Design review of the part built by this model. Coordinates are the model's own, in mm. A direction names the side the tool comes from. Coordinates: 2 decimals unless noted, no trailing zeros. Write each loop counter-clockwise with the first axis right and the second up, starting at its lowest first coordinate (ties: lowest second). Pieces come first, ordered by that corner, then holes. Notation, with made-up numbers: (76.5, 77.25) - (84.5, 77.25) arc R16 ccw to (84.5, 108.25) - close; hole circle Ø5 at (5, 60.25). An arc over 180 degrees is marked (long way). Use a Markdown table: item, result.
from build123d import *

# Parameters (mm, degrees)
F0_W           = 5.9
F0_H           = 1.1
F1_DEPTH       = 2.9
F2_W           = 5.9
F2_H           = 1.85
F3_DEPTH       = 2
F5_D           = 3.2
F5_CSINK_D     = 5.6
F5_CSINK_ANGLE = 82
F6_DEPTH       = 1.1
F7_R           = 1
F8_W           = 3
F8_H           = 1.2
F9_DEPTH       = 2.6
F10_W          = 1.6
F10_H          = 2.7
F10_H_2        = 1.55
F11_DEPTH      = 3.5
F12_W          = 1.6
F12_H          = 1.35
F13_DEPTH      = 1.6
F15_DEPTH      = 2.8


with BuildPart() as f1:
    # F0 (on Top) → F1 (new body)
    with BuildSketch(Plane.XY):
        with BuildLine():
            Line((4.95, 1.6), (4.95, 0))
            Line((4.95, 0), (12.45, 0))
            Line((12.45, 0), (12.45, 1.6))
            Line((12.45, 1.6), (15.45, 1.6))
            Line((15.45, 1.6), (15.45, 0))
            Line((15.45, 0), (19.3, 0))
            Line((19.3, 0), (19.3, 1.1))
            Line((19.3, 1.1), (25.2, 1.1))
            Line((25.2, 1.1), (25.2, 0))
            Line((25.2, 0), (29.05, 0))
            Line((29.05, 0), (29.05, 1.6))
            Line((29.05, 1.6), (32.05, 1.6))
            Line((32.05, 1.6), (32.05, 0))
            Line((32.05, 0), (39.55, 0))
            Line((39.55, 0), (39.55, 1.6))
            Line((39.55, 1.6), (42.55, 1.6))
            Line((42.55, 1.6), (42.55, 0))
            Line((42.55, 0), (42.7, 0))
            ThreePointArc((42.7, 0), (43.9727922061, 0.5272077939), (44.5, 1.8))
            Line((44.5, 1.8), (44.5, 42.7))
            ThreePointArc((44.5, 42.7), (43.9727922061, 43.9727922061), (42.7, 44.5))
            Line((42.7, 44.5), (42.55, 44.5))
            Line((42.55, 44.5), (42.55, 42.9))
            Line((42.55, 42.9), (39.55, 42.9))
            Line((39.55, 42.9), (39.55, 44.5))
            Line((39.55, 44.5), (32.05, 44.5))
            Line((32.05, 44.5), (32.05, 42.9))
            Line((32.05, 42.9), (29.05, 42.9))
            Line((29.05, 42.9), (29.05, 44.5))
            Line((29.05, 44.5), (25.2, 44.5))
            Line((25.2, 44.5), (25.2, 43.4))
            Line((25.2, 43.4), (19.3, 43.4))
            Line((19.3, 43.4), (19.3, 44.5))
            Line((19.3, 44.5), (15.45, 44.5))
            Line((15.45, 44.5), (15.45, 42.9))
            Line((15.45, 42.9), (12.45, 42.9))
            Line((12.45, 42.9), (12.45, 44.5))
            Line((12.45, 44.5), (4.95, 44.5))
            Line((4.95, 44.5), (4.95, 42.9))
            Line((4.95, 42.9), (1.95, 42.9))
            Line((1.95, 42.9), (1.95, 44.5))
            Line((1.95, 44.5), (1.8, 44.5))
            ThreePointArc((1.8, 44.5), (0.5272077939, 43.9727922061), (0, 42.7))
            Line((0, 42.7), (0, 1.8))
            ThreePointArc((0, 1.8), (0.5272077939, 0.5272077939), (1.8, 0))
            Line((1.8, 0), (1.95, 0))
            Line((1.95, 0), (1.95, 1.6))
            Line((1.95, 1.6), (4.95, 1.6))
        make_face()
        with Locations((22.25, -0.55)):
            Rectangle(F0_W, F0_H)
        with Locations((22.25, 0.55)):
            Rectangle(F0_W, F0_H)
        with Locations((22.25, 43.95)):
            Rectangle(F0_W, F0_H)
        with Locations((22.25, 45.05)):
            Rectangle(F0_W, F0_H)
    extrude(amount=F1_DEPTH)

    # F2 (on face) → F3 (join)
    with BuildSketch(Plane(origin=(0, 0, 0), x_dir=(1, 0, 0), z_dir=(0, 0, -1))):
        with Locations((22.25, 0.175)):
            Rectangle(F2_W, F2_H)
        with BuildLine():
            Line((25.2, -0.75), (19.3, -0.75))
            Line((19.3, -0.75), (9.7372574326, -2.4247745488))
            ThreePointArc((9.7372574326, -2.4247745488), (4.9258838609, -4.9258838609), (2.4247745488, -9.7372574326))
            Line((2.4247745488, -9.7372574326), (0.75, -19.3))
            Line((0.75, -19.3), (0.75, -25.2))
            Line((0.75, -25.2), (2.4247745488, -34.7627425674))
            ThreePointArc((2.4247745488, -34.7627425674), (4.9258838609, -39.5741161391), (9.7372574326, -42.0752254512))
            Line((9.7372574326, -42.0752254512), (19.3, -43.75))
            Line((19.3, -43.75), (25.2, -43.75))
            Line((25.2, -43.75), (34.7627425674, -42.0752254512))
            ThreePointArc((34.7627425674, -42.0752254512), (39.5741161391, -39.5741161391), (42.0752254512, -34.7627425674))
            Line((42.0752254512, -34.7627425674), (43.75, -25.2))
            Line((43.75, -25.2), (43.75, -19.3))
            Line((43.75, -19.3), (42.0752254512, -9.7372574326))
            ThreePointArc((42.0752254512, -9.7372574326), (39.5741161391, -4.9258838609), (34.7627425674, -2.4247745488))
            Line((34.7627425674, -2.4247745488), (25.2, -0.75))
        make_face()
        with Locations((22.25, -44.675)):
            Rectangle(F2_W, F2_H)
    extrude(amount=F3_DEPTH)

    # F5 (through all)
    with Locations(Plane.XY.offset(2.9)):
        with Locations((22.25, 41.25), (22.25, 3.25)):
            CounterSinkHole(F5_D / 2, F5_CSINK_D / 2, counter_sink_angle=F5_CSINK_ANGLE)

    # F6 (add): a face of the model
    f6_faces = [f1.faces().sort_by_distance(p)[0] for p in [
        (22.25, 22.25, 2.9),
    ]]
    extrude(f6_faces, amount=F6_DEPTH)

    # F7
    f7_edges = [f1.edges().sort_by_distance(p)[0] for p in [
        (25.2, -1.1, 1),
        (19.3, -1.1, 1),
        (25.2, 45.6, 1),
        (19.3, 45.6, 1),
    ]]
    fillet(f7_edges, radius=F7_R)

    # F8 (on face) → F9 (cut, through all)
    with BuildSketch(Plane(origin=(0, 0, 0), x_dir=(1, 0, 0), z_dir=(0, 0, -1))):
        with Locations((3.45, -42.3)):
            Rectangle(F8_W, F8_H)
        with Locations((13.95, -42.3)):
            Rectangle(F8_W, F8_H)
        with Locations((3.45, -2.2)):
            Rectangle(F8_W, F8_H)
        with Locations((13.95, -2.2)):
            Rectangle(F8_W, F8_H)
        with Locations((30.55, -42.3)):
            Rectangle(F8_W, F8_H)
        with Locations((41.05, -42.3)):
            Rectangle(F8_W, F8_H)
        with Locations((30.55, -2.2)):
            Rectangle(F8_W, F8_H)
        with Locations((41.05, -2.2)):
            Rectangle(F8_W, F8_H)
    extrude(amount=-F9_DEPTH, mode=Mode.SUBTRACT)

    # F10 (on face) → F11 (cut)
    with BuildSketch(Plane.XY.offset(4)):
        Polygon((19.25, 1.55), (19.25, 4.25), (17.65, 4.25), (17.65, 1.55), (17.65, 0), (19.25, 0), align=None)
        with Locations((18.45, 41.6)):
            Rectangle(F10_W, F10_H)
        with Locations((18.45, 43.725)):
            Rectangle(F10_W, F10_H_2)
        Polygon((25.25, 4.25), (25.25, 1.55), (25.25, 0), (26.85, 0), (26.85, 1.55), (26.85, 4.25), align=None)
        Polygon((25.25, 42.95), (25.25, 40.25), (26.85, 40.25), (26.85, 42.95), (26.85, 44.5), (25.25, 44.5), align=None)
    extrude(amount=-F11_DEPTH, mode=Mode.SUBTRACT)

    # F12 (on face) → F13 (join)
    with BuildSketch(Plane.XY.offset(4)):
        with Locations((26.05, 0.675)):
            Rectangle(F12_W, F12_H)
        with Locations((18.45, 0.675)):
            Rectangle(F12_W, F12_H)
        with Locations((26.05, 43.825)):
            Rectangle(F12_W, F12_H)
        with Locations((18.45, 43.825)):
            Rectangle(F12_W, F12_H)
    extrude(amount=-F13_DEPTH)

    # F14 (on face) → F15 (cut, through all)
    with BuildSketch(Plane.XY.offset(4)):
        with BuildLine():
            Line((16.45, 40.5), (1.2, 40.5))
            Line((1.2, 40.5), (1.2, 22.25))
            Line((1.2, 22.25), (1.2, 4))
            Line((1.2, 4), (16.45, 4))
            Line((16.45, 4), (16.45, 5.45))
            Line((16.45, 5.45), (18.9093410611, 5.45))
            ThreePointArc((18.9093410611, 5.45), (22.25, 7.2500002682), (25.5906589389, 5.45))
            Line((25.5906589389, 5.45), (28.05, 5.45))
            Line((28.05, 5.45), (28.05, 4))
            Line((28.05, 4), (43.3, 4))
            Line((43.3, 4), (43.3, 22.25))
            Line((43.3, 22.25), (43.3, 40.5))
            Line((43.3, 40.5), (28.05, 40.5))
            Line((28.05, 40.5), (28.05, 39.05))
            Line((28.05, 39.05), (25.5906589389, 39.05))
            ThreePointArc((25.5906589389, 39.05), (22.25, 37.2499997318), (18.9093410611, 39.05))
            Line((18.9093410611, 39.05), (16.45, 39.05))
            Line((16.45, 39.05), (16.45, 40.5))
        make_face()
    extrude(amount=-F15_DEPTH, mode=Mode.SUBTRACT)


solid = f1.part
(1) Take a section at D-D on x = 4. Write out the cut boundary in (y, z), and give its area (3 significant figures).
Determined:
| item | result |
|---|---|
| outline | (1.6, 2.6) - (2.8, 2.6) - (2.8, 0) - (6.01, 0) - (6.01, -2) - (38.49, -2) - (38.49, 0) - (41.7, 0) - (41.7, 2.6) - (42.9, 2.6) - (42.9, 4) - (40.5, 4) - (40.5, 1.2) - (4, 1.2) - (4, 4) - (1.6, 4) - close |
| area | 122 mm2 |
(2) Take a section at C-C on x = 38.5. Write out the cut boundary in (y, z).
Determined:
| item | result |
|---|---|
| outline | (0, 0) - (4.01, 0) - (4.01, -2) - (40.49, -2) - (40.49, 0) - (44.5, 0) - (44.5, 4) - (40.5, 4) - (40.5, 1.2) - (4, 1.2) - (4, 4) - (0, 4) - close |
(3) Machinability: for faces 4 (the flat face through (25.25, 3, 2)), 5 (the flat face through (42.55, 43, 2)), 6 (the flat face through (1.95, 1, 2)), 7 (the flat face through (28, 44.5, 2)), which of the approach directions +Z, -Z, +X, -X, +Y, -Y give a long, thin tool a straight path to every point of the face, cutting with its end or side? Answer none if there is none.
Determined:
| item | result |
|---|---|
| face 4 | none |
| face 5 | -Z, +Y |
| face 6 | -Z, -Y |
| face 7 | +Z, -Z, +X, +Y |
(4) Draft analysis for pull direction X (two halves, no side actions). For faces 1 (the flat face through (22, 22, -2)), 2 (the flat face through (30.05, 1.6, -0.99)), 3 (the flat face through (31, 2, 2.6)), state which applies: +X half, -X half, draft (parallel to the pull), parting line (faces both ways), or undercut.
Determined:
| item | result |
|---|---|
| face 1 | draft |
| face 2 | +X half |
| face 3 | undercut |
(5) For pin 1 (2 mm diameter, centred on x = 40.5, z = 1, fed in from +Y); pin 2 (1.3 mm diameter, centred on x = 30, z = 1, fed in from +Y); pin 3 (5 mm diameter, centred on x = 30, y = 13.5, fed in from +Z); pin 4 (3.5 mm diameter, centred on x = 22.25, y = 41.25, fed in from -Z), all flat-tipped, find the tip position at first contact; note any pin that passes through.
Determined:
| item | result |
|---|---|
| pin 1 | y = 44.5 |
| pin 2 | y = 41.7 |
| pin 3 | z = 1.2 |
| pin 4 | z = -2 |
(6) Take a section at A-A on x = 22.25. Write out the cut boundary in (y, z).
Determined:
| item | result |
|---|---|
| outline | (-1.1, -2) - (1.65, -2) - (1.65, 1.52) - (0.45, 2.9) - (0.45, 4) - (-1.1, 4) - close; (4.85, -2) - (39.65, -2) - (39.65, 1.52) - (38.45, 2.9) - (38.45, 4) - (37.25, 4) - (37.25, 1.2) - (7.25, 1.2) - (7.25, 4) - (6.05, 4) - (6.05, 2.9) - (4.85, 1.52) - close; (42.85, -2) - (45.6, -2) - (45.6, 4) - (44.05, 4) - (44.05, 2.9) - (42.85, 1.52) - close |
(7) For L1, parallel to Y at x = 22.25, z = 3.8; L2, parallel to Y at x = 22.25, z = -0.7; L3, parallel to X at y = 41.25, z = -0.15, list the stretches that pass through material, from the lowest coordinate up. Write a range as from..to.
Determined:
| item | result |
|---|---|
| L1 | -1.1..0.45, 6.05..7.25, 37.25..38.45, 44.05..45.6 |
| L2 | -1.1..1.65, 4.85..39.65, 42.85..45.6 |
| L3 | 7.24..20.65, 23.85..37.26 |
(8) Take a section at B-B on y = 34. Write out the cut boundary in (x, z), and give its area (3 significant figures).
Determined:
| item | result |
|---|---|
| outline | (0, 0) - (2.29, 0) - (2.29, -2) - (42.21, -2) - (42.21, 0) - (44.5, 0) - (44.5, 4) - (43.3, 4) - (43.3, 1.2) - (1.2, 1.2) - (1.2, 4) - (0, 4) - close |
| area | 140 mm2 |
